Design review of the part built by this model. Coordinates are the model's own, in mm. Round coordinates to 2 decimals unless told otherwise and drop trailing zeros. Loops run counter-clockwise (first coordinate to the right, second up) from the corner with the lowest first, then second, coordinate; pieces in that order, holes last. Notation, with made-up numbers: (22.5, 34.5) - (46.5, 34.5) arc R25 cw to (46.5, 72.5) - close; hole circle Ø2 at (85, 9.25). An arc over 180 degrees is marked (long way). Use one line per item in the form item = value. Start each with the question number.
(1) Wall thickness on probe 1 along Y at (x, z) = (0, 15.5); probe 2 along X at (y, z) = (-3, 30.5); probe 3 along Y at (x, z) = (4.5, 17): over which ranges is each line inside the solid? List them lowest first. Write a range as [from, to].
(2) We need section D-D, the plane x = 16.5. Write out the cut boundary in (y, z).
(3) We need section B-B, the plane x = 0. Write out the cut boundary in (y, z).
(4) We need section C-C, the plane z = 25.5. Write out the cut boundary in (x, y).
(5) We need section A-A, the plane y = 0. Write out the cut boundary in (x, z), then the cut area to 3 significant figures.
(6) The part is to be moulded in two halves that separate along Y. For faces 1 (the cylindrical face through (-5.5, -24.9, 17.3)), 2 (the flat face through (11, 0, 0)), 3 (the cylindrical face through (20.5, 0.1, 17.3)), say which applies: released by +Y, released by -Y, zero draft, split by the parting line, or undercut.
(7) For pin 1 (4.5 mm diameter, centred on y = -17, z = 22, fed in from +X); pin 2 (5 mm diameter, centred on y = -9.5, z = 19, fed in from -X); pin 3 (12 mm diameter, centred on y = 2.5, z = 21.5, fed in from +X); pin 4 (9.5 mm diameter, centred on y = 17, z = 13, fed in from +X), all flat-tipped, find the tip position at first contact; note any pin that passes through.
from build123d import *

# Parameters (mm, degrees)
ESQUISSE1_R      = 25.5
ESQUISSE1_R_2    = 9.5
EXTRUSION1_DEPTH = 35


with BuildPart() as part:
    # Esquisse1 → Extrusion1 (new body)
    with BuildSketch(Plane.XY):
        Circle(ESQUISSE1_R)
        Circle(ESQUISSE1_R_2, mode=Mode.SUBTRACT)
        with BuildLine():
            Line((10.856157589, 5.113104968), (18.232385626, 9.371772211))
            ThreePointArc((18.232385626, 9.371772211), (20.5, 0), (18.232385626, -9.371772211))
            Line((18.232385626, -9.371772211), (10.856157589, -5.113104968))
            ThreePointArc((10.856157589, -5.113104968), (12, 0), (10.856157589, 5.113104968))
        make_face(mode=Mode.SUBTRACT)
        with BuildLine():
            Line((9.856157589, 6.845155775), (17.232385626, 11.103823019))
            ThreePointArc((17.232385626, 11.103823019), (10.25, 17.753520778), (1, 20.475595229))
            Line((1, 20.475595229), (1, 11.958260743))
            ThreePointArc((1, 11.958260743), (6, 10.392304845), (9.856157589, 6.845155775))
        make_face(mode=Mode.SUBTRACT)
        with BuildLine():
            Line((9.856157589, -6.845155775), (17.232385626, -11.103823019))
            ThreePointArc((17.232385626, -11.103823019), (10.25, -17.753520778), (1, -20.475595229))
            Line((1, -20.475595229), (1, -11.958260743))
            ThreePointArc((1, -11.958260743), (6, -10.392304845), (9.856157589, -6.845155775))
        make_face(mode=Mode.SUBTRACT)
        with BuildLine():
            Line((-1, 11.958260743), (-1, 20.475595229))
            ThreePointArc((-1, 20.475595229), (-10.25, 17.753520778), (-17.232385626, 11.103823019))
            Line((-17.232385626, 11.103823019), (-9.856157589, 6.845155775))
            ThreePointArc((-9.856157589, 6.845155775), (-6, 10.392304845), (-1, 11.958260743))
        make_face(mode=Mode.SUBTRACT)
        with BuildLine():
            Line((-1, -11.958260743), (-1, -20.475595229))
            ThreePointArc((-1, -20.475595229), (-10.25, -17.753520778), (-17.232385626, -11.103823019))
            Line((-17.232385626, -11.103823019), (-9.856157589, -6.845155775))
            ThreePointArc((-9.856157589, -6.845155775), (-6, -10.392304845), (-1, -11.958260743))
        make_face(mode=Mode.SUBTRACT)
        with BuildLine():
            Line((-10.856157589, -5.113104968), (-18.232385626, -9.371772211))
            ThreePointArc((-18.232385626, -9.371772211), (-20.5, 0), (-18.232385626, 9.371772211))
            Line((-18.232385626, 9.371772211), (-10.856157589, 5.113104968))
            ThreePointArc((-10.856157589, 5.113104968), (-12, 0), (-10.856157589, -5.113104968))
        make_face(mode=Mode.SUBTRACT)
    extrude(amount=EXTRUSION1_DEPTH)


solid = part.part
Data:
q1.probe_1 = [-25.5, -9.5], [9.5, 25.5]
q1.probe_2 = [-25.32, -20.28], [-11.62, -9.01], [9.01, 11.62], [20.28, 25.32]
q1.probe_3 = [-25.1, -20], [-11.12, -8.37], [8.37, 11.12], [20, 25.1]
q2.outline = (-19.44, 0) - (-12.17, 0) - (-12.17, 35) - (-19.44, 35) - close; (-10.68, 0) - (-8.37, 0) - (-8.37, 35) - (-10.68, 35) - close; (8.37, 0) - (10.68, 0) - (10.68, 35) - (8.37, 35) - close; (12.17, 0) - (19.44, 0) - (19.44, 35) - (12.17, 35) - close
q3.outline = (-25.5, 0) - (-9.5, 0) - (-9.5, 35) - (-25.5, 35) - close; (9.5, 0) - (25.5, 0) - (25.5, 35) - (9.5, 35) - close
q4.outline = circle Ø51 at (0, 0); hole (-18.23, -9.37) - (-10.86, -5.11) arc R12 cw to (-10.86, 5.11) - (-18.23, 9.37) arc R20.5 ccw to start; hole (-17.23, -11.1) arc R20.5 ccw to (-1, -20.48) - (-1, -11.96) arc R12 cw to (-9.86, -6.85) - close; hole (-17.23, 11.1) - (-9.86, 6.85) arc R12 cw to (-1, 11.96) - (-1, 20.48) arc R20.5 ccw to start; hole circle Ø19 at (0, 0); hole (1, -20.48) arc R20.5 ccw to (17.23, -11.1) - (9.86, -6.85) arc R12 cw to (1, -11.96) - close; hole (1, 11.96) arc R12 cw to (9.86, 6.85) - (17.23, 11.1) arc R20.5 ccw to (1, 20.48) - close; hole (10.86, -5.11) - (18.23, -9.37) arc R20.5 ccw to (18.23, 9.37) - (10.86, 5.11) arc R12 cw to start
q5.outline = (-25.5, 0) - (-20.5, 0) - (-20.5, 35) - (-25.5, 35) - close; (-12, 0) - (-9.5, 0) - (-9.5, 35) - (-12, 35) - close; (9.5, 0) - (12, 0) - (12, 35) - (9.5, 35) - close; (20.5, 0) - (25.5, 0) - (25.5, 35) - (20.5, 35) - close
q5.area = 525 mm^2
q6.face_1 = split by the parting line
q6.face_2 = zero draft
q6.face_3 = undercut
q7.pin_1 = 20.8
q7.pin_2 = -24.52
q7.pin_3 = 25.5
q7.pin_4 = 22.36
